```python
from build123d import *

# Parameters (mm, degrees)
SKETCH1_R           = 2.75
BOSS_EXTRUDE1_DEPTH = 5.207


with BuildPart() as part:
    # Sketch1 → Boss-Extrude1 (new body)
    with BuildSketch(Plane.XY):
        Polygon((-189.357, 25.4), (-189.357, 0), (-157.607, 0), (-157.607, 330.2), (157.607, 330.2), (157.607, 0), (189.357, 0), (189.357, 25.4), (184.15, 25.4), (184.15, 50.8), (189.357, 50.8), (189.357, 76.2), (184.15, 76.2), (184.15, 101.6), (189.357, 101.6), (189.357, 127), (184.15, 127), (184.15, 152.4), (189.357, 152.4), (189.357, 177.8), (184.15, 177.8), (184.15, 203.2), (189.357, 203.2), (189.357, 228.6), (184.15, 228.6), (184.15, 254), (189.357, 254), (189.357, 279.4), (184.15, 279.4), (184.15, 304.8), (189.357, 304.8), (189.357, 330.2), (184.15, 330.2), (184.15, 355.6), (189.357, 355.6), (189.357, 381), (184.15, 381), (184.15, 406.4), (-184.15, 406.4), (-184.15, 381), (-189.357, 381), (-189.357, 355.6), (-184.15, 355.6), (-184.15, 330.2), (-189.357, 330.2), (-189.357, 304.8), (-184.15, 304.8), (-184.15, 279.4), (-189.357, 279.4), (-189.357, 254), (-184.15, 254), (-184.15, 228.6), (-189.357, 228.6), (-189.357, 203.2), (-184.15, 203.2), (-184.15, 177.8), (-189.357, 177.8), (-189.357, 152.4), (-184.15, 152.4), (-184.15, 127), (-189.357, 127), (-189.357, 101.6), (-184.15, 101.6), (-184.15, 76.2), (-189.357, 76.2), (-189.357, 50.8), (-184.15, 50.8), (-184.15, 25.4), align=None)
        with Locations((-171.45, 368.05)):
            Circle(SKETCH1_R, mode=Mode.SUBTRACT)
        with Locations((-171.45, 400.05)):
            Circle(SKETCH1_R, mode=Mode.SUBTRACT)
        with Locations((171.45, 368.05)):
            Circle(SKETCH1_R, mode=Mode.SUBTRACT)
        with Locations((171.45, 400.05)):
            Circle(SKETCH1_R, mode=Mode.SUBTRACT)
    extrude(amount=BOSS_EXTRUDE1_DEPTH)


solid = part.part
```
Design review of the part built by this model. Coordinates are the model's own, in mm. Give positions to 0.01 mm unless a question says otherwise; leave off trailing zeros. Write each loop counter-clockwise with the first axis right and the second up, starting at its lowest first coordinate (ties: lowest second). Pieces come first, ordered by that corner, then holes. Notation, with made-up numbers: (7.5, 27.5) - (27.5, 27.5) arc R8 cw to (27.5, 36.5) - close; hole circle Ø6 at (69.25, 72). An arc over 180 degrees is marked (long way). Return JSON: item names as keys, results as strings. Group by question number.
(1) To check wall thickness, follow probe 1 along Y at (x, z) = (171.45, 1.4); probe 2 along X at (y, z) = (400.05, 3.35); probe 3 along X at (y, z) = (368.05, 2.25). State the ranges of each line that lie inside material, in increasing order.
(2) We need section C-C, the plane z = 3.4. Give the number of separate pieces and of enclosed holes in the cut face, then the cut area to 3 significant figures.
(3) We need section A-A, the plane y = 92.5. Give the boundary of the cut face in (x, z), then the cut area to 3 significant figures.
(4) Insertion check: pin 1 (2.5 mm diameter, centred on y = 190.5, z = 2.5, fed in from -X); pin 2 (1.6 mm diameter, centred on x = -187, z = 2.5, fed in from +Y); pin 3 (2.5 mm diameter, centred on x = 187.5, z = 1.5, fed in from -Y); pin 4 (3.5 mm diameter, centred on x = -171.45, y = 400.05, fed in from +Z). Each pin has a flat end and moves straight along its axis. Give the tip position at first contact, or say it passes through.
(5) We need section D-D, the plane x = 57. Give the boundary of the cut face in (y, z), then the cut area to 3 significant figures.
(6) We need section B-B, the plane y = 170. Give the boundary of the cut face in (x, z), then the cut area to 3 significant figures.
Reported:
{
 "1": {"probe 1": "y = 0 to 365.3, 370.8 to 397.3, 402.8 to 406.4", "probe 2": "x = -184.15 to -174.2, -168.7 to 168.7, 174.2 to 184.15", "probe 3": "x = -189.36 to -174.2, -168.7 to 168.7, 174.2 to 189.36"},
 "2": {"separate pieces": "1", "enclosed holes": "4", "area": "47,600 mm2"},
 "3": {"outline": "(-184.15, 0) - (-157.61, 0) - (-157.61, 5.21) - (-184.15, 5.21) - close; (157.61, 0) - (184.15, 0) - (184.15, 5.21) - (157.61, 5.21) - close", "area": "276 mm2"},
 "4": {"pin 1": "stops at x = -184.15", "pin 2": "stops at y = 381", "pin 3": "stops at y = 0", "pin 4": "passes through"},
 "5": {"outline": "(330.2, 0) - (406.4, 0) - (406.4, 5.21) - (330.2, 5.21) - close", "area": "397 mm2"},
 "6": {"outline": "(-189.36, 0) - (-157.61, 0) - (-157.61, 5.21) - (-189.36, 5.21) - close; (157.61, 0) - (189.36, 0) - (189.36, 5.21) - (157.61, 5.21) - close", "area": "331 mm2"}
}
